from build123d import *

# Parameters (mm, degrees)
F0_R     = 10.95
F1_DEPTH = 2.4
F2_R     = 4.035
F3_DEPTH = 4.2
F4_R     = 1
F5_R     = 5.2
F5_R_2   = 4.035
F6_DEPTH = 0.7
F7_R     = 1
F8_R     = 8
F9_DEPTH = 1
F11_SIZE = 0.6
F12_R    = 6


# Not quite as in the source:
# - a fillet or chamfer that OpenCascade refuses, or shapes differently, is made with other operations: its cross-section is extruded or revolved along the edge and cut away or added


with BuildPart() as f1:
    # F0 (on Top) → F1 (new body)
    with BuildSketch(Plane.XY):
        Circle(F0_R)
    extrude(amount=F1_DEPTH)

    # F2 (on face) → F3 (join)
    with BuildSketch(Plane.XY.offset(2.4)):
        Circle(F2_R)
    extrude(amount=F3_DEPTH)

    # F4
    f4_edges = [f1.edges().sort_by_distance(p)[0] for p in [
        (-10.95, 0, 2.4),
    ]]
    fillet(f4_edges, radius=F4_R)

    # F5 (on face) → F6 (join)
    with BuildSketch(Plane.XY.offset(2.4)):
        Circle(F5_R)
        Circle(F5_R_2, mode=Mode.SUBTRACT)
    extrude(amount=F6_DEPTH)

    # F7
    f7_edges = [f1.edges().sort_by_distance(p)[0] for p in [
        (-10.95, 0, 0),
    ]]
    fillet(f7_edges, radius=F7_R)

    # F8 (on face) → F9 (cut)
    with BuildSketch(Plane(origin=(0, 0, 0), x_dir=(1, 0, 0), z_dir=(0, 0, -1))):
        Circle(F8_R)
    extrude(amount=-F9_DEPTH, mode=Mode.SUBTRACT)

    # F10: fillet of radius 11 on 1 edges, made by hand

    # F10_s1 → F10_t2 (revolve)
    with BuildSketch(Plane.XZ):
        with BuildLine():
            ThreePointArc((8, 0), (5.762632185, 0.7470926301), (3.417424305, 1))
            Line((3.417424305, 1), (8, 1))
            Line((8, 1), (8, 0))
        make_face()
    revolve(axis=Axis((0, 0, 1), (0, 0, -1)))

    # F11
    f11_edges = [f1.edges().sort_by_distance(p)[0] for p in [
        (-4.035, 0, 6.6),
    ]]
    chamfer(f11_edges, length=F11_SIZE)

    # F12
    f12_edges = [f1.edges().sort_by_distance(p)[0] for p in [
        (-8, 0, 0),
    ]]
    fillet(f12_edges, radius=F12_R)


solid = f1.part
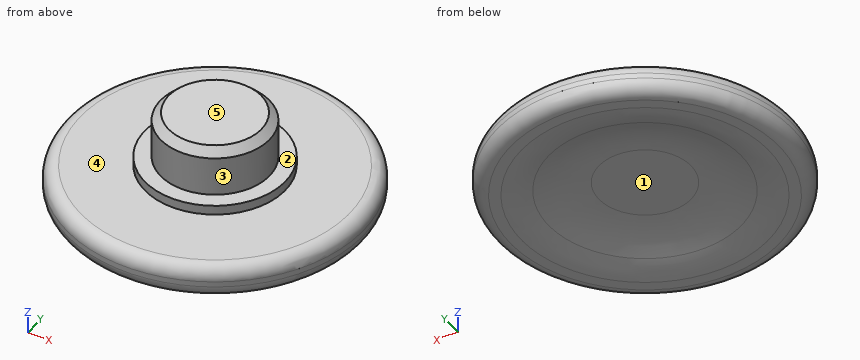
Source: CAD feature listing. Evaluate the final solid. Frame: model axes, mm. Face numbers are marked on the shaded views. A direction names the side the tool comes from. Round coordinates to 2 decimals unless told otherwise and drop trailing zeros. Loops run counter-clockwise (first coordinate to the right, second up) from the corner with the lowest first, then second, coordinate; pieces in that order, holes last.
Q1. Mould query, pull axis X, two halves, no side actions, for the marked faces 1, 2 and 3. Classes: pulls with the +X half, pulls with the -X half, needs draft (parallel to the pull), parting line crosses it, or undercut.
Q2. Access query for the marked faces 4 and 5. Directions: +Z, -Z, +X, -X, +Y, -Y. A direction counts if a zero-diameter tool reaches every point of the face in a straight line with its end or side. Return the directions, or none.
Q3. First-contact query: P1, Ø8, axis at x = 0.5, y = 3, coming from the -Z side; P2, Ø3, axis at x = -8, y = -6, coming from the +Z side; P3, Ø5.5, axis at x = 0.5, y = 0, coming from the -Z side. Flat tips, straight axial feed; report the tip coordinate or a pass-through.
Q4. Section A-A, the plane z = 3.75. Return loops of the section in (x, y) (3 decimals), plus the area to 3 significant figures.
Q5. Ray query, line 1 (Z direction, x = -1, y = -1); line 2 (Z direction, x = -2.25, y = 4); line 3 (Y direction, x = -1.5, z = 3.75). Return the intervals inside material, ascending.
Solutions:
1. face 1: undercut
1. face 2: needs draft
1. face 3: parting line crosses it
2. face 4: +Z
2. face 5: +Z, +X, -X, +Y, -Y
3. P1: stops at z = 0.39
3. P2: stops at z = 2.4
3. P3: stops at z = 1
4. outline: circle Ø8.07 at (0, 0)
4. area: 51.1 mm2
5. line 1: z = 1 to 6.6
5. line 2: z = 0.94 to 3.1
5. line 3: y = -3.75 to 3.75
